from build123d import *

# Parameters (mm, degrees)
BOSS_EXTRUDE1_DEPTH = 2
SKETCH2_R           = 2.5
SKETCH2_R_2         = 1
BOSS_EXTRUDE2_DEPTH = 13
BOSS_EXTRUDE3_DEPTH = 7.5


with BuildPart() as part:
    # Sketch1 → Boss-Extrude1 (new body)
    with BuildSketch(Plane(origin=(0, 0, 0), x_dir=(1, 0, 0), z_dir=(0, 1, 0))):
        with BuildLine():
            Line((0.858370189, 99.070664528), (76.558370189, 99.070664528))
            ThreePointArc((76.558370189, 99.070664528), (78.679690533, 98.191984872), (79.558370189, 96.070664528))
            Line((79.558370189, 96.070664528), (79.558370189, 1.370664528))
            ThreePointArc((79.558370189, 1.370664528), (78.679690533, -0.750655815), (76.558370189, -1.629335472))
            Line((76.558370189, -1.629335472), (0.858370189, -1.629335472))
            ThreePointArc((0.858370189, -1.629335472), (-1.262950154, -0.750655815), (-2.141629811, 1.370664528))
            Line((-2.141629811, 1.370664528), (-2.141629811, 96.070664528))
            ThreePointArc((-2.141629811, 96.070664528), (-1.262950154, 98.191984872), (0.858370189, 99.070664528))
        make_face()
    extrude(amount=BOSS_EXTRUDE1_DEPTH)

    # Sketch2 → Boss-Extrude2 (add)
    # profile 1 of 4: a face of its own
    with BuildSketch(Plane(origin=(0, 2, 0), x_dir=(1, 0, 0), z_dir=(0, 1, 0))):
        with Locations(Location((10.381260955, 10.570783491, 0), (0, 0, 90))):
            Circle(SKETCH2_R)
        with Locations(Location((10.381260955, 10.570783491, 0), (0, 0, 90))):
            Circle(SKETCH2_R_2, mode=Mode.SUBTRACT)
    # profile 2 of 4: a face of its own
    with BuildSketch(Plane(origin=(0, 2, 0), x_dir=(1, 0, 0), z_dir=(0, 1, 0))):
        with Locations(Location((67.381260955, 6.770783491, 0), (0, 0, 90))):
            Circle(SKETCH2_R)
        with Locations(Location((67.381260955, 6.770783491, 0), (0, 0, 90))):
            Circle(SKETCH2_R_2, mode=Mode.SUBTRACT)
    # profile 3 of 4: a face of its own
    with BuildSketch(Plane(origin=(0, 2, 0), x_dir=(1, 0, 0), z_dir=(0, 1, 0))):
        with Locations(Location((60.731260955, 86.570783491, 0), (0, 0, 90))):
            Circle(SKETCH2_R)
        with Locations(Location((60.731260955, 86.570783491, 0), (0, 0, 90))):
            Circle(SKETCH2_R_2, mode=Mode.SUBTRACT)
    # profile 4 of 4: a face of its own
    with BuildSketch(Plane(origin=(0, 2, 0), x_dir=(1, 0, 0), z_dir=(0, 1, 0))):
        with Locations(Location((36.981260955, 77.070783491, 0), (0, 0, 90))):
            Circle(SKETCH2_R)
        with Locations(Location((36.981260955, 77.070783491, 0), (0, 0, 90))):
            Circle(SKETCH2_R_2, mode=Mode.SUBTRACT)
    extrude(amount=BOSS_EXTRUDE2_DEPTH)

    # Sketch3 → Boss-Extrude3 (add)
    with BuildSketch(Plane(origin=(0, 2, 0), x_dir=(1, 0, 0), z_dir=(0, 1, 0))):
        with BuildLine():
            Line((76.744157469, 98.956147889), (1.044157469, 98.956147889))
            ThreePointArc((1.044157469, 98.956147889), (-1.077162875, 98.077468232), (-1.955842531, 95.956147889))
            Line((-1.955842531, 95.956147889), (-1.955842531, 1.256147889))
            ThreePointArc((-1.955842531, 1.256147889), (-1.601404378, -0.158420071), (-0.621840855, -1.238736795))
            ThreePointArc((-0.621840855, -1.238736795), (0.092930436, -1.530042624), (0.858370189, -1.629335472))
            Line((0.858370189, -1.629335472), (76.558370189, -1.629335472))
            ThreePointArc((76.558370189, -1.629335472), (78.679690533, -0.750655815), (79.558370189, 1.370664528))
            Line((79.558370189, 1.370664528), (79.558370189, 96.070664528))
            ThreePointArc((79.558370189, 96.070664528), (79.203932036, 97.485232488), (78.224368514, 98.565549212))
            ThreePointArc((78.224368514, 98.565549212), (77.509597222, 98.856855041), (76.744157469, 98.956147889))
        make_face()
        with BuildLine():
            ThreePointArc((0.044157469, 95.956147889), (0.337050688, 96.66325467), (1.044157469, 96.956147889))
            Line((1.044157469, 96.956147889), (76.744157469, 96.956147889))
            ThreePointArc((76.744157469, 96.956147889), (77.45126425, 96.66325467), (77.744157469, 95.956147889))
            Line((77.744157469, 95.956147889), (77.744157469, 1.256147889))
            ThreePointArc((77.744157469, 1.256147889), (77.45126425, 0.549041108), (76.744157469, 0.256147889))
            Line((76.744157469, 0.256147889), (1.044157469, 0.256147889))
            ThreePointArc((1.044157469, 0.256147889), (0.337050688, 0.549041108), (0.044157469, 1.256147889))
            Line((0.044157469, 1.256147889), (0.044157469, 95.956147889))
        make_face(mode=Mode.SUBTRACT)
    extrude(amount=BOSS_EXTRUDE3_DEPTH)


solid = part.part
Input: part model. Units: mm. Frame: model coordinates. A direction names the side the tool comes from. Round coordinates to 2 decimals unless told otherwise and drop trailing zeros. Loops run counter-clockwise (first coordinate to the right, second up) from the corner with the lowest first, then second, coordinate; pieces in that order, holes last. Notation, with made-up numbers: M 23,-3 L 38,-3 A23 cw 38,20 Z; hole C 13.25,50.25 d5. An arc over 180 degrees is marked long. Answer as CSV lines item,"result". Start each with the question number.
(1) Section C-C, the plane x = 43.5. Output: boundary loops of the cut face in (y, z).
(2) Section B-B, the plane z = -53. Output: boundary loops of the cut face in (x, y).
(3) Section A-A, the plane y = 11. Output: boundary loops of the cut face in (x, z).
(4) Draft query along Z for faces 1 (the flat face through (39, 6, -98.956)), 2 (the cylindrical face through (60.621, 8.409, -84.073)), 3 (the cylindrical face through (-1.61, 5.7, 0.14)). Return one class per face: released by +Z, released by -Z, zero draft, split by the parting line, or undercut.
(5) Line query: line 1 (Z direction, x = 17, y = 2.25); line 2 (X direction, y = 7, z = -54); line 3 (X direction, y = 13.25, z = -77). Output: solid intervals per line, ascending. Write a range as [from, to].
(6) First-contact query: pin 1 (8 mm diameter, centred on x = 31.5, y = 11, fed in from -Z); pin 2 (4 mm diameter, centred on y = 5.5, z = -78.5, fed in from -X); pin 3 (1.2 mm diameter, centred on x = 60.73, z = -86.57, fed in from +Y); pin 4 (3 mm diameter, centred on x = 67.38, z = -6.77, fed in from -Y). Flat tips, straight axial feed; report the tip coordinate or a pass-through.
(7) Reachability of faces 4 (the flat face through (67, 15, -8)), 5 (the cylindrical face through (-1.054, 5.698, -98.101)), 6 (the flat face through (61, 2, -87)) from +Z, -Z, +X, -X, +Y, -Y: full face, straight path, thin tool, end or side. Return the list, or none.
Values found:
1,outline,"M 0,-99.07 L 2,-99.07 L 2,-98.96 L 9.5,-98.96 L 9.5,-96.96 L 2,-96.96 L 2,-0.26 L 9.5,-0.26 L 9.5,1.63 L 0,1.63 Z"
2,outline,"M -2.14,0 L 79.56,0 L 79.56,9.5 L 77.74,9.5 L 77.74,2 L 0.04,2 L 0.04,9.5 L -1.96,9.5 L -1.96,2 L -2.14,2 Z"
3,outline,"C 10.38,-10.57 d5; C 36.98,-77.07 d5; C 60.73,-86.57 d5; C 67.38,-6.77 d5; hole C 10.38,-10.57 d2; hole C 36.98,-77.07 d2; hole C 60.73,-86.57 d2; hole C 67.38,-6.77 d2"
4,face 1,"released by -Z"
4,face 2,"undercut"
4,face 3,"released by +Z"
5,line 1,"z = [-98.96, -96.96], [-0.26, 1.63]"
5,line 2,"x = [-1.96, 0.04], [77.74, 79.56]"
5,line 3,"x = [34.48, 35.98], [37.98, 39.48]"
6,pin 1,"stops at z = -98.96"
6,pin 2,"stops at x = -1.96"
6,pin 3,"stops at y = 2"
6,pin 4,"stops at y = 0"
7,face 4,"+Z, -Z, +X, -X, +Y"
7,face 5,"-Z, -X, +Y"
7,face 6,"+Y"
